from build123d import *

# Parameters (mm, degrees)
SKETCH1_W               = 9.525
SKETCH1_H               = 19.05
BOSS_EXTRUDE1_DEPTH     = 6.35
CUT_EXTRUDE4_DEPTH      = 15.892070037
CUT_EXTRUDE4_DEPTH_BACK = 15.892070037
CUT_EXTRUDE6_DEPTH      = 11.962309672
CUT_EXTRUDE6_DEPTH_BACK = 11.962309672
SKETCH7_R               = 2.54
FILLET2_R               = 0.79375
FILLET3_R               = 0.15875


with BuildPart() as part:
    # Sketch1 → Boss-Extrude1 (new body)
    with BuildSketch(Plane(origin=(0, 0, 0), x_dir=(1, 0, 0), z_dir=(0, 1, 0))):
        Rectangle(SKETCH1_W, SKETCH1_H)
    extrude(amount=BOSS_EXTRUDE1_DEPTH)

    # Sketch4 → Cut-Extrude4 (cut, two sides: drawn at the far end of the back side and taken through both)
    with BuildSketch(Plane.ZY.offset(4.7625).offset(-CUT_EXTRUDE4_DEPTH_BACK)):
        Polygon((9.525, 0.311917294), (-9.525, 3.56560647), (-9.525, 6.35), (9.525, 6.35), align=None)
    extrude(amount=CUT_EXTRUDE4_DEPTH + CUT_EXTRUDE4_DEPTH_BACK, mode=Mode.SUBTRACT)

    # Sketch7 → Cut-Extrude6 (cut, two sides: drawn at the far end of the back side and taken through both)
    with BuildSketch(Plane(origin=(0, 1.911087398, 0.162031127), x_dir=(1, 0, 0), z_dir=(0, -0.9857256920245803, -0.16835931837193446)).offset(-CUT_EXTRUDE6_DEPTH_BACK)):
        with Locations(Location((0, -3.914374553, 0), (0, 0, 270))):
            Circle(SKETCH7_R)
    extrude(amount=CUT_EXTRUDE6_DEPTH + CUT_EXTRUDE6_DEPTH_BACK, mode=Mode.SUBTRACT)

    # Fillet2
    # the kernel refuses this fillet: 0.79375 mm, written as the material it takes off along each edge
    with BuildSketch(Plane(origin=(3.96875, 0.79375, -8.73125), x_dir=(1, 0, 0), z_dir=(0, -1, 0))) as fillet2_piece_1_section:
        Polygon((0, 0), (FILLET2_R, 0), (FILLET2_R, -FILLET2_R), (0, -FILLET2_R), align=None)
    fillet2_piece_1 = extrude(amount=FILLET2_R, mode=Mode.PRIVATE)
    fillet2_piece_1 = fillet2_piece_1 - Plane(origin=(3.96875, 0.79375, -8.73125), x_dir=(-0.7071067811865475, 0, 0.7071067811865475), z_dir=(0, -1, 0)) * Sphere(FILLET2_R, mode=Mode.PRIVATE)
    add(fillet2_piece_1, mode=Mode.SUBTRACT)
    with BuildSketch(Plane(origin=(3.96875, 2.624791783, -8.73125), x_dir=(0, 0.9857256920245803, 0.16835931837193446), z_dir=(1, 0, 0))) as fillet2_piece_2_section:
        Polygon((0, 0), (FILLET2_R, 0), (FILLET2_R, -FILLET2_R * 1.18527834653), (-FILLET2_R * 0.168359318372, -FILLET2_R * 0.985725692025), align=None)
    fillet2_piece_2 = extrude(amount=FILLET2_R, mode=Mode.PRIVATE)
    fillet2_piece_2 = fillet2_piece_2 - Plane(origin=(3.96875, 2.624791783, -8.73125), x_dir=(0, -0.7643164653374722, 0.6448413299518206), z_dir=(1, 0, 0)) * Sphere(FILLET2_R, mode=Mode.PRIVATE)
    add(fillet2_piece_2, mode=Mode.SUBTRACT)
    with BuildSketch(Plane(origin=(-3.96875, 0.79375, -8.73125), x_dir=(-1, 0, 0), z_dir=(0, -1, 0))) as fillet2_piece_3_section:
        Polygon((0, 0), (FILLET2_R, 0), (FILLET2_R, FILLET2_R), (0, FILLET2_R), align=None)
    fillet2_piece_3 = extrude(amount=FILLET2_R, mode=Mode.PRIVATE)
    fillet2_piece_3 = fillet2_piece_3 - Plane(origin=(-3.96875, 0.79375, -8.73125), x_dir=(0.7071067811865475, 0, 0.7071067811865475), z_dir=(0, -1, 0)) * Sphere(FILLET2_R, mode=Mode.PRIVATE)
    add(fillet2_piece_3, mode=Mode.SUBTRACT)
    with BuildSketch(Plane(origin=(-3.96875, 2.624791783, -8.73125), x_dir=(0, 0, -1), z_dir=(-1, 0, 0))) as fillet2_piece_4_section:
        Polygon((0, 0), (FILLET2_R, 0), (FILLET2_R, -FILLET2_R * 1.18527834653), (-FILLET2_R * 0.168359318372, -FILLET2_R * 0.985725692025), align=None)
    fillet2_piece_4 = extrude(amount=FILLET2_R, mode=Mode.PRIVATE)
    fillet2_piece_4 = fillet2_piece_4 - Plane(origin=(-3.96875, 2.624791783, -8.73125), x_dir=(0, -0.7643164653374722, 0.6448413299518206), z_dir=(-1, 0, 0)) * Sphere(FILLET2_R, mode=Mode.PRIVATE)
    add(fillet2_piece_4, mode=Mode.SUBTRACT)
    with BuildSketch(Plane(origin=(4.7625, 0, 11.509375), x_dir=(-1, 0, 0), z_dir=(0, 0, -1)), Plane(origin=(-4.7625, 0, -8.73125), x_dir=(1, 0, 0), z_dir=(0, 0, 1))) as fillet2_piece_5:
        with BuildLine():
            CenterArc((FILLET2_R, FILLET2_R), FILLET2_R, 180, 90)
            Line((0, FILLET2_R), (0, 0))
            Line((0, 0), (FILLET2_R, 0))
        make_face()
    extrude(amount=20.240625, mode=Mode.SUBTRACT)
    with BuildSketch(Plane(origin=(4.7625, 3.407211551, -8.597614791), x_dir=(0, -0.9857256920245803, -0.16835931837193446), z_dir=(0, -0.16835931837193446, 0.9857256920245803))) as fillet2_piece_6:
        with BuildLine():
            CenterArc((FILLET2_R, -FILLET2_R), FILLET2_R, 90, 90)
            Line((0, -FILLET2_R), (0, 0))
            Line((0, 0), (FILLET2_R, 0))
        make_face()
    extrude(amount=20.369423637, mode=Mode.SUBTRACT)
    with BuildSketch(Plane(origin=(3.96875, 0, -9.525), x_dir=(0, 0, 1), z_dir=(-1, 0, 0))) as fillet2_piece_7:
        with BuildLine():
            CenterArc((FILLET2_R, FILLET2_R), FILLET2_R, 180, 90)
            Line((0, FILLET2_R), (0, 0))
            Line((0, 0), (FILLET2_R, 0))
        make_face()
    extrude(amount=7.9375, mode=Mode.SUBTRACT)
    with BuildSketch(Plane(origin=(4.7625, 0.79375, -9.525), x_dir=(0, 0, 1), z_dir=(0, 1, 0))) as fillet2_piece_8:
        with BuildLine():
            CenterArc((FILLET2_R, -FILLET2_R), FILLET2_R, 90, 90)
            Line((0, -FILLET2_R), (0, 0))
            Line((0, 0), (FILLET2_R, 0))
        make_face()
    extrude(amount=1.831041783, mode=Mode.SUBTRACT)
    with BuildSketch(Plane(origin=(-3.96875, 3.56560647, -9.525), x_dir=(0, -0.16835931837193435, 0.9857256920245803), z_dir=(1, 0, 0))) as fillet2_piece_9:
        with BuildLine():
            CenterArc((FILLET2_R * 1.18527834653, FILLET2_R), FILLET2_R, 170.307559955, 99.692440045)
            Line((FILLET2_R * 0.199552654502, FILLET2_R * 1.16835931837), (0, 0))
            Line((0, 0), (FILLET2_R * 1.18527834653, 0))
        make_face()
    extrude(amount=7.9375, mode=Mode.SUBTRACT)
    with BuildSketch(Plane(origin=(-4.7625, 0.79375, -9.525), x_dir=(0, 0, 1), z_dir=(0, 1, 0))) as fillet2_piece_10:
        with BuildLine():
            CenterArc((FILLET2_R, FILLET2_R), FILLET2_R, 180, 90)
            Line((0, FILLET2_R), (0, 0))
            Line((0, 0), (FILLET2_R, 0))
        make_face()
    extrude(amount=1.831041783, mode=Mode.SUBTRACT)
    with BuildSketch(Plane(origin=(-4.7625, -0.022170729, 11.48104942), x_dir=(1, 0, 0), z_dir=(0, 0.16835931837193446, -0.9857256920245803))) as fillet2_piece_11:
        with BuildLine():
            CenterArc((FILLET2_R, FILLET2_R), FILLET2_R, 180, 90)
            Line((0, FILLET2_R), (0, 0))
            Line((0, 0), (FILLET2_R, 0))
        make_face()
    extrude(amount=20.369423637, mode=Mode.SUBTRACT)

    # Fillet3
    fillet3_edges = [part.edges().sort_by_distance(p)[0] for p in [
        (-4.216643426, 0.039702314, 9.525),
        (4.216643426, 0.039702314, 9.525),
        (4.216960585, 0.271534198, 9.525),
        (-4.216960585, 0.271534198, 9.525),
        (0, 0, 9.525),
        (0, 0.311917294, 9.525),
    ]]
    fillet(fillet3_edges, radius=FILLET3_R)


solid = part.part
Geometry check sheet. Reference: the model listing, model coordinates, mm. Give positions to 0.01 mm unless a question says otherwise; leave off trailing zeros. Answer in a Markdown table with one row per item. Add a question column.
1) Draft check along Z on faces 1 (the face through (0.76, 1.83, -6.28)), 2 (the face through (-4.762, 1, -6)), 3 (the face through (0, 2, -9.525)), 4 (the face through (4.5, 1.7, 0.2)). Enter one of: pulls with the +Z half, pulls with the -Z half, needs draft (parallel to the pull), parting line crosses it, or undercut.
2) Gauge pin test, flat end, axial feed: P1, Ø3, axis at x = -2.5, z = 4, coming from the +Y side. Record the tip position at first contact, or that the pin passes through.
3) Material ranges on probe 1 along X at (y, z) = (0.85, -3.75); probe 2 along Y at (x, z) = (1.25, 3); probe 3 along Y at (x, z) = (0.75, 6.25), recorded low to high. Write a range as from..to.
Outcome:
| question | item | result |
|---|---|---|
| 1 | face 1 | undercut |
| 1 | face 2 | needs draft |
| 1 | face 3 | pulls with the -Z half |
| 1 | face 4 | pulls with the +Z half |
| 2 | P1 | stops at y = 1.51 |
| 3 | probe 1 | x = -4.76..-2.53, 2.53..4.76 |
| 3 | probe 2 | y = 0..1.43 |
| 3 | probe 3 | y = 0..0.87 |
